Autodesk Fusion 360 part; units mm, degrees
sketch "Sketch1" plane through (0, 0, 0) normal (1, 0, 0) x (0, 1, 0)
  line L0 (20, -24) -> (-20, -24)
  line L1 (-20, -24) -> (-20, 4)
  line L2 (20, 4) -> (20, -24)
  arc A0 (20, 4) -> (-20, 4) centre (0, 4) ccw
  line L3 (-6.25, 4) -> (-6.25, -15)
  arc A1 (-6.25, -15) -> (6.25, -15) centre (0, -15) ccw
  line L4 (6.25, -15) -> (6.25, 4)
  arc A2 (6.25, 4) -> (-6.25, 4) centre (0, 4) ccw
  line L5 (0, 4) -> (0, -15) construction
  circle A3 centre (-16.237, 4) radius 1.6
  circle A4 centre (-10, -20) radius 1.6
  circle A5 centre (10, -20) radius 1.6
  circle A6 centre (-10, 10) radius 1.6
  circle A7 centre (10, 10) radius 1.6
  circle A8 centre (16.237, 4) radius 1.6
  dimension "d4" = 12.5
  dimension "d5" = 3.2
  dimension "d6" = 3.2
  dimension "d9" = 20
  dimension "d10" = 30
extrude "Extrude1" add sketch "Sketch1" along normal blind 1.5
sketch "Sketch2" plane through (0, 0, 0) normal (-1, 0, 0) x (0, -1, 0)
  circle A0 centre (10, 10) radius 1.6
  circle A1 centre (-10, 10) radius 1.6
  circle A2 centre (-16.237, 4) radius 1.6
  circle A3 centre (10, -20) radius 1.6
  circle A4 centre (-10, -20) radius 1.6
  circle A5 centre (16.237, 4) radius 1.6
  arc A6 (6.25, 4) -> (-6.25, 4) centre (0, 4) ccw
  line L0 (6.25, 4) -> (6.25, -15)
  arc A7 (-6.25, -15) -> (6.25, -15) centre (0, -15) ccw
  line L1 (-6.25, -15) -> (-6.25, 4)
  line L2 (-20, 4) -> (-20, -24)
  line L3 (-20, -24) -> (20, -24)
  line L4 (20, -24) -> (20, 4)
  arc A8 (20, 4) -> (-20, 4) centre (0, 4) ccw
  line L5 (-20, -24) -> (20, -24)
  line L6 (20, -24) -> (20, -22.5)
  line L7 (20, -22.5) -> (-20, -22.5)
  line L8 (-20, -22.5) -> (-20, -24)
  dimension "d13" = 1.5
extrude "Extrude2" add sketch "Sketch2" along normal blind 30 contours L2 L3 L4 L5 L6 L7 L8
sketch "Sketch3" plane through (0, 0, -22.5) normal (0, 0, 1) x (-1, 0, 0)
  line L0 (0, 20) -> (0, -20)
  line L1 (0, -20) -> (30, -20)
  line L2 (30, -20) -> (30, 20)
  line L3 (30, 20) -> (0, 20)
sketch "Sketch4" plane through (0, 0, -22.5) normal (0, 0, 1) x (1, 0, 0)
  line L0 (-23.5, 12.9) -> (-9.5, 12.9)
  arc A0 (-9.5, 12.9) -> (-9.5, 17.1) centre (-9.5, 15) ccw
  line L1 (-9.5, 17.1) -> (-23.5, 17.1)
  arc A1 (-23.5, 17.1) -> (-23.5, 12.9) centre (-23.5, 15) ccw
  line L2 (-23.5, 15) -> (-9.5, 15) construction
  line L3 (-23.5, -12.9) -> (-9.5, -12.9)
  arc A2 (-23.5, -12.9) -> (-23.5, -17.1) centre (-23.5, -15) ccw
  line L4 (-9.5, -17.1) -> (-23.5, -17.1)
  arc A3 (-9.5, -17.1) -> (-9.5, -12.9) centre (-9.5, -15) ccw
  line L5 (-26.2852, 7.0901) -> (-26.2852, -6.9099)
  arc A4 (-26.2852, -6.9099) -> (-22.0852, -6.9099) centre (-24.1852, -6.9099) ccw
  line L6 (-22.0852, -6.9099) -> (-22.0852, 7.0901)
  arc A5 (-22.0852, 7.0901) -> (-26.2852, 7.0901) centre (-24.1852, 7.0901) ccw
  line L7 (-24.1852, 7.0901) -> (-24.1852, -6.9099) construction
  line L8 (-7.9148, -6.9099) -> (-7.9148, 7.0901)
  arc A6 (-3.7148, 7.0901) -> (-7.9148, 7.0901) centre (-5.8148, 7.0901) ccw
  line L9 (-3.7148, 7.0901) -> (-3.7148, -6.9099)
  arc A7 (-7.9148, -6.9099) -> (-3.7148, -6.9099) centre (-5.8148, -6.9099) ccw
  dimension "d17" = 14
  dimension "d18" = 4.2
  dimension "d19" = 4.2
extrude "Extrude3" cut sketch "Sketch4" against normal blind 1.5
The model under review builds one solid part; all positions refer to its coordinate system, in mm. A direction names the side the tool comes from. Coordinates: 2 decimals unless noted, no trailing zeros. Write each loop counter-clockwise with the first axis right and the second up, starting at its lowest first coordinate (ties: lowest second). Pieces come first, ordered by that corner, then holes. Notation, with made-up numbers: (63.25, -21.75) - (109.25, -21.75) arc R15 ccw to (109.25, -5.75) - close; hole circle Ø5 at (63.5, 55). An arc over 180 degrees is marked (long way). Answer in a Markdown table with one row per item. Add a question column.
Q1. Consider section A-A on z = 1.5. Give the boundary of the cut face in (x, y).
Q2. Draft analysis for pull direction Z (two halves, no side actions). For faces 1 (the face through (1.5, 9, 0)), 2 (the face through (0.74, -14.71, 3.52)), 3 (the face through (-15, 0, -22.5)), state which applies: +Z half, -Z half, draft (parallel to the pull), parting line (faces both ways), or undercut.
Q3. Consider section B-B on x = -17.5. Give the boundary of the cut face in (y, z).
Q4. For faces 4 (the face through (0.74, -0.14, 10.25)), 5 (the face through (-14, 0, -24)), 6 (the face through (-3.715, 0, -23)), 7 (the face through (0, -9, 1)), 8 (the face through (-30, 0, -23)), list the 3-axis set-ups (+Z, -Z, +X, -X, +Y, -Y) from which the entire face can be reached by the end or side of a thin tool; tool diameter is ignored.
Q5. Consider section C-C on y = 10.5. Give the boundary of the cut face in (x, z).
Q6. To check wall thickness, follow line 1 along Z through (x, y) = (0.8, -10); line 2 along X through (y, z) = (5.5, 9); line 3 along Z through (x, y) = (-11, -3.5). State the ranges of each line that lie inside material, in increasing order. Write a range as from..to.
Q7. Clearance check with flat-ended pins moving along their axes: pin 1 (9 mm diameter, centred on x = -15.5, y = -1, fed in from +Z); pin 2 (3 mm diameter, centred on y = 8.5, z = -5, fed in from -X). State where each tip first meets the part, or that it passes through.
Q8. Consider section D-D on x = -3. Give the boundary of the cut face in (y, z).
Answers below:
| question | item | result |
|---|---|---|
| 1 | outline | (0, -20) - (1.5, -20) - (1.5, -6.25) - (0, -6.25) - close; (0, 6.25) - (1.5, 6.25) - (1.5, 20) - (0, 20) - close |
| 2 | face 1 | draft |
| 2 | face 2 | undercut |
| 2 | face 3 | +Z half |
| 3 | outline | (-20, -24) - (-17.1, -24) - (-17.1, -22.5) - (-20, -22.5) - close; (-12.9, -24) - (12.9, -24) - (12.9, -22.5) - (-12.9, -22.5) - close; (17.1, -24) - (20, -24) - (20, -22.5) - (17.1, -22.5) - close |
| 4 | face 4 | +X, -X |
| 4 | face 5 | -Z, +X, -X, +Y, -Y |
| 4 | face 6 | +Z, -Z |
| 4 | face 7 | +Z, -X, +Y, -Y |
| 4 | face 8 | +Z, -Z, -X, +Y, -Y |
| 5 | outline | (-30, -24) - (1.5, -24) - (1.5, -21.52) - (0, -21.52) - (0, -22.5) - (-30, -22.5) - close; (0, -18.48) - (1.5, -18.48) - (1.5, 8.48) - (0, 8.48) - close; (0, 11.52) - (1.5, 11.52) - (1.5, 21.02) - (0, 21.02) - close |
| 6 | line 1 | -24..-21.6, -18.4..8.4, 11.6..21.32 |
| 6 | line 2 | 0..1.5 |
| 6 | line 3 | -24..-22.5 |
| 7 | pin 1 | z = -22.5 |
| 7 | pin 2 | x = 0 |
| 8 | outline | (-20, -24) - (20, -24) - (20, -22.5) - (-20, -22.5) - close |
